Read the model definition and answer for the solid it produces. Units are mm, in the model's axes. A direction names the side the tool comes from. Coordinates: 2 decimals unless noted, no trailing zeros. Write each loop counter-clockwise with the first axis right and the second up, starting at its lowest first coordinate (ties: lowest second). Pieces come first, ordered by that corner, then holes. Notation, with made-up numbers: (-18.75, 85.25) -> (26.25, 85.25) arc R27 ccw to (26.25, 121.25) -> close; hole circle Ø3 at (36, 33.25). An arc over 180 degrees is marked (long way). Write item = value, one per line. Start each with the question number.
1) Section B-B (z = 12.25) is taken. Determine the outline of the cut face in (x, y).
2) Find the intervals of material crossed by line 1 along Z through (x, y) = (-30.5, 1.6); line 2 along Z through (x, y) = (-9, 4); line 3 along X through (y, z) = (2.55, 8.25), in increasing order. Write a range as from..to.
3) Section A-A (y = 2.2) is taken. Determine the outline of the cut face in (x, z), plus the area to 3 significant figures.
4) Flat-ended cylindrical pins translate along their axes: pin 1 Ø1 at (x, y) = (17.5, 3.5) entering from +Z; pin 2 Ø3 at (x, y) = (-10.5, 1.5) entering from +Z; pin 3 Ø2.5 at (y, z) = (4, 12) entering from -X. Find the tip coordinate at first contact, or state that the pin passes through.
5) A tool of negligible diameter and unlimited length cuts with its end or side. For faces 1 (the face through (-27.5, 3, 8)), 2 (the face through (22, 3, 10)), 3 (the face through (-27.5, 3, -7)), from which of +Z, -Z, +X, -X, +Y, -Y can it reach the whole face along a straight path? Write none if from no direction.
6) Section C-C (x = 2) is taken. Determine the outline of the cut face in (y, z), plus the area to 3 significant figures.
from build123d import *

# Parameters (mm, degrees)
SKETCH1_W              = 55
SKETCH1_H              = 20
BOSS_EXTRUDE1_DEPTH    = 6
SKETCH234_W            = 10
SKETCH234_H            = 6
BOSS_EXTRUDE234_DEPTH  = 6
FILLET134_R            = 1
SKETCH2342_W           = 10
SKETCH2342_H           = 6
BOSS_EXTRUDE2342_DEPTH = 6
FILLET1342_R           = 1
FILLET1343_R           = 5


with BuildPart() as part:
    # Sketch1 → Boss-Extrude1 (new body)
    with BuildSketch(Plane(origin=(0, 0, 0), x_dir=(1, 0, 0), z_dir=(0, 1, 0))):
        Rectangle(SKETCH1_W, SKETCH1_H)
    extrude(amount=BOSS_EXTRUDE1_DEPTH)

    # Sketch234 → Boss-Extrude234 (add)
    with BuildSketch(Plane(origin=(13.267778608, 6, 10), x_dir=(-1, 0, 0), z_dir=(0, 0, 1))):
        with Locations((0.767778608, 3)):
            Rectangle(SKETCH234_W, SKETCH234_H)
    extrude(amount=BOSS_EXTRUDE234_DEPTH)

    # Fillet134
    fillet134_edges = [part.edges().sort_by_distance(p)[0] for p in [
        (17.5, 3, 16),
        (7.5, 3, 16),
    ]]
    fillet(fillet134_edges, radius=FILLET134_R)

    # Sketch2342 → Boss-Extrude2342 (add)
    with BuildSketch(Plane(origin=(-27.5, 0, -0.767778608), x_dir=(0, 0, 1), z_dir=(-1, 0, 0))):
        with Locations((0.767778608, 3)):
            Rectangle(SKETCH2342_W, SKETCH2342_H)
    extrude(amount=BOSS_EXTRUDE2342_DEPTH)

    # Fillet1342
    fillet1342_edges = [part.edges().sort_by_distance(p)[0] for p in [
        (-33.5, 3, -5),
        (-33.5, 3, 5),
    ]]
    fillet(fillet1342_edges, radius=FILLET1342_R)

    # Fillet1343
    fillet1343_edges = [part.edges().sort_by_distance(p)[0] for p in [
        (27.5, 3, -10),
    ]]
    fillet(fillet1343_edges, radius=FILLET1343_R)


solid = part.part
Answer key:
q1.outline = (7.5, 0) -> (17.5, 0) -> (17.5, 6) -> (7.5, 6) -> close
q2.line_1 = -5..5
q2.line_2 = -10..10
q2.line_3 = -27.5..27.5
q3.outline = (-33.5, -4) arc R1 ccw to (-32.5, -5) -> (-27.5, -5) -> (-27.5, -10) -> (22.5, -10) arc R5 ccw to (27.5, -5) -> (27.5, 10) -> (17.5, 10) -> (17.5, 15) arc R1 ccw to (16.5, 16) -> (8.5, 16) arc R1 ccw to (7.5, 15) -> (7.5, 10) -> (-27.5, 10) -> (-27.5, 5) -> (-32.5, 5) arc R1 ccw to (-33.5, 4) -> close
q3.area = 1,210 mm^2
q4.pin_1 = 15.87
q4.pin_2 = 10
q4.pin_3 = 7.5
q5.face_1 = +Z, -X, +Y, -Y
q5.face_2 = +Z, +X, +Y, -Y
q5.face_3 = -Z, -X, +Y, -Y
q6.outline = (0, -10) -> (6, -10) -> (6, 10) -> (0, 10) -> close
q6.area = 120 mm^2
